For this review, take the finished solid that the model builds, in its own axes (mm). A direction names the side the tool comes from. Give positions to 0.01 mm unless a question says otherwise; leave off trailing zeros. Use a Markdown table: item, result. Add a question column.
1) Machinability: for faces 1 (the face through (1.972, 219.188, -129.733)), 2 (the face through (0, 118, -125)), which of the approach directions +Z, -Z, +X, -X, +Y, -Y give a long, thin tool a straight path to every point of the face, cutting with its end or side? Answer none if there is none.
2) Wall thickness on L1, parallel to Y at x = 1.15, z = -177.8; L2, parallel to Y at x = 2, z = -139.7; L3, parallel to Y at x = 2.4, z = -79: over which ranges is each line inside the solid? List them lowest first.
3) Mouldability with a two-part tool opening along Z and no side actions: class faces 3 (the face through (1.972, 212.884, -126.987)), 4 (the face through (4, 118, -125)), 5 (the face through (1.97, 225.77, -125.22)) as released by +Z, released by -Z, zero draft, split by the parting line, or undercut.
4) Clearance check with a flat-ended pin moving along its axis: P1, Ø8, axis at y = 12.7, z = -215.9, coming from the -X side. State where the tip first meets the part, or that it passes through.
5) We need section A-A on x = 2.05. Give the number of separate pieces and of enclosed holes in the cut face, then the cut area to 3 significant figures.
Autodesk Inventor part; units mm, degrees
ref_plane "YZ Plane" through (0, 0, 0) normal (1, 0, 0) x (0, 1, 0)
ref_plane "XZ Plane" through (0, 0, 0) normal (0, 1, 0) x (-1, 0, 0)
ref_plane "XY Plane" through (0, 0, 0) normal (0, 0, 1) x (1, 0, 0)
sketch "Esboço1" plane through (0, 0, 0) normal (1, 0, 0) x (0, 1, 0)
  line L0 (0, 0) -> (203.2, 0)
  line L1 (203.2, 0) -> (228.6, -254)
  line L2 (228.6, -254) -> (0, -254)
  line L3 (0, -254) -> (0, 0)
  circle A0 centre (12.7, 0) radius 2.5
  circle A1 centre (25.4, 0) radius 2.5
  circle A2 centre (38.1, 0) radius 2.5
  circle A3 centre (38.1, -12.7) radius 2.5
  circle A4 centre (25.4, -12.7) radius 2.5
  circle A5 centre (12.7, -12.7) radius 2.5
  circle A6 centre (38.1, -25.4) radius 2.5
  circle A7 centre (25.4, -25.4) radius 2.5
  circle A8 centre (12.7, -25.4) radius 2.5
  circle A9 centre (38.1, -38.1) radius 2.5
  circle A10 centre (25.4, -38.1) radius 2.5
  circle A11 centre (12.7, -38.1) radius 2.5
  circle A12 centre (38.1, -50.8) radius 2.5
  circle A13 centre (25.4, -50.8) radius 2.5
  circle A14 centre (12.7, -50.8) radius 2.5
  circle A15 centre (38.1, -63.5) radius 2.5
  circle A16 centre (25.4, -63.5) radius 2.5
  circle A17 centre (12.7, -63.5) radius 2.5
  circle A18 centre (38.1, -76.2) radius 2.5
  circle A19 centre (25.4, -76.2) radius 2.5
  circle A20 centre (12.7, -76.2) radius 2.5
  circle A21 centre (38.1, -88.9) radius 2.5
  circle A22 centre (25.4, -88.9) radius 2.5
  circle A23 centre (12.7, -88.9) radius 2.5
  circle A24 centre (38.1, -101.6) radius 2.5
  circle A25 centre (25.4, -101.6) radius 2.5
  circle A26 centre (12.7, -101.6) radius 2.5
  circle A27 centre (38.1, -114.3) radius 2.5
  circle A28 centre (25.4, -114.3) radius 2.5
  circle A29 centre (12.7, -114.3) radius 2.5
  circle A30 centre (38.1, -127) radius 2.5
  circle A31 centre (25.4, -127) radius 2.5
  circle A32 centre (12.7, -127) radius 2.5
  circle A33 centre (38.1, -139.7) radius 2.5
  circle A34 centre (25.4, -139.7) radius 2.5
  circle A35 centre (12.7, -139.7) radius 2.5
  circle A36 centre (38.1, -152.4) radius 2.5
  circle A37 centre (25.4, -152.4) radius 2.5
  circle A38 centre (12.7, -152.4) radius 2.5
  circle A39 centre (38.1, -165.1) radius 2.5
  circle A40 centre (25.4, -165.1) radius 2.5
  circle A41 centre (12.7, -165.1) radius 2.5
  circle A42 centre (38.1, -177.8) radius 2.5
  circle A43 centre (25.4, -177.8) radius 2.5
  circle A44 centre (12.7, -177.8) radius 2.5
  circle A45 centre (38.1, -190.5) radius 2.5
  circle A46 centre (25.4, -190.5) radius 2.5
  circle A47 centre (12.7, -190.5) radius 2.5
  circle A48 centre (38.1, -203.2) radius 2.5
  circle A49 centre (25.4, -203.2) radius 2.5
  circle A50 centre (12.7, -203.2) radius 2.5
  circle A51 centre (38.1, -215.9) radius 2.5
  circle A52 centre (25.4, -215.9) radius 2.5
  circle A53 centre (12.7, -215.9) radius 2.5
  circle A54 centre (38.1, -228.6) radius 2.5
  circle A55 centre (25.4, -228.6) radius 2.5
  circle A56 centre (12.7, -228.6) radius 2.5
  circle A57 centre (38.1, -241.3) radius 2.5
  circle A58 centre (25.4, -241.3) radius 2.5
  circle A59 centre (12.7, -241.3) radius 2.5
  circle A60 centre (38.1, -254) radius 2.5
  circle A61 centre (25.4, -254) radius 2.5
  circle A62 centre (12.7, -254) radius 2.5
  circle A63 centre (203.4985, -2.9851) radius 3
  circle A64 centre (204.0955, -8.9553) radius 3
  circle A65 centre (204.6926, -14.9256) radius 3
  circle A66 centre (205.2896, -20.8958) radius 3
  circle A67 centre (205.8866, -26.866) radius 3
  circle A68 centre (206.4836, -32.8362) radius 3
  circle A69 centre (207.0806, -38.8065) radius 3
  circle A70 centre (207.6777, -44.7767) radius 3
  circle A71 centre (208.2747, -50.7469) radius 3
  circle A72 centre (208.8717, -56.7171) radius 3
  circle A73 centre (209.4687, -62.6873) radius 3
  circle A74 centre (210.0658, -68.6576) radius 3
  circle A75 centre (210.6628, -74.6278) radius 3
  circle A76 centre (211.2598, -80.598) radius 3
  circle A77 centre (211.8568, -86.5682) radius 3
  circle A78 centre (212.4538, -92.5385) radius 3
  circle A79 centre (213.0509, -98.5087) radius 3
  circle A80 centre (213.6479, -104.4789) radius 3
  circle A81 centre (214.2449, -110.4491) radius 3
  circle A82 centre (214.8419, -116.4194) radius 3
  circle A83 centre (215.439, -122.3896) radius 3
  circle A84 centre (216.036, -128.3598) radius 3
  circle A85 centre (216.633, -134.33) radius 3
  circle A86 centre (217.23, -140.3002) radius 3
  circle A87 centre (217.827, -146.2705) radius 3
  circle A88 centre (218.4241, -152.2407) radius 3
  circle A89 centre (219.0211, -158.2109) radius 3
  circle A90 centre (219.6181, -164.1811) radius 3
  circle A91 centre (220.2151, -170.1514) radius 3
  circle A92 centre (220.8122, -176.1216) radius 3
  circle A93 centre (221.4092, -182.0918) radius 3
  circle A94 centre (222.0062, -188.062) radius 3
  circle A95 centre (222.6032, -194.0323) radius 3
  circle A96 centre (223.2002, -200.0025) radius 3
  circle A97 centre (223.7973, -205.9727) radius 3
  circle A98 centre (224.3943, -211.9429) radius 3
  circle A99 centre (224.9913, -217.9131) radius 3
  circle A100 centre (225.5883, -223.8834) radius 3
  circle A101 centre (226.1854, -229.8536) radius 3
  circle A102 centre (226.7824, -235.8238) radius 3
  circle A103 centre (227.3794, -241.794) radius 3
  circle A104 centre (227.9764, -247.7643) radius 3
  circle A105 centre (228.5734, -253.7345) radius 3
  line L4 (203.2, 0) -> (213.2499, 0)
  line L5 (213.2499, 0) -> (238.6499, -254)
  line L6 (238.6499, -254) -> (228.6, -254)
  line L7 (227.9764, -247.7643) -> (204.0955, -8.9553) construction
  line L8 (230.9615, -247.4657) -> (207.0806, -8.6568)
  line L9 (201.1104, -9.2538) -> (224.9913, -248.0628)
  arc A106 (224.9913, -248.0628) -> (230.9615, -247.4657) centre (227.9764, -247.7643) ccw
  arc A107 (207.0806, -8.6568) -> (201.1104, -9.2538) centre (204.0955, -8.9553) ccw
  point P0 (40.6, 0)
  point P1 (35.6, 0)
  point P2 (27.9, 0)
  point P3 (22.9, 0)
  point P4 (15.2, 0)
  point P5 (10.2, 0)
  point P6 (10.2, -254)
  point P7 (15.2, -254)
  point P8 (22.9, -254)
  point P9 (27.9, -254)
  point P10 (35.6, -254)
  point P11 (40.6, -254)
  point P12 (203.797, -5.9702)
  point P13 (204.394, -11.9404)
  point P14 (204.9911, -17.9107)
  point P15 (205.5881, -23.8809)
  point P16 (206.1851, -29.8511)
  point P17 (206.7821, -35.8213)
  point P18 (207.3792, -41.7916)
  point P19 (207.9762, -47.7618)
  point P20 (208.5732, -53.732)
  point P21 (209.1702, -59.7022)
  point P22 (209.7672, -65.6725)
  point P23 (210.3643, -71.6427)
  point P24 (210.9613, -77.6129)
  point P25 (211.5583, -83.5831)
  point P26 (212.1553, -89.5533)
  point P27 (212.7524, -95.5236)
  point P28 (213.3494, -101.4938)
  point P29 (213.9464, -107.464)
  point P30 (214.5434, -113.4342)
  point P31 (215.1404, -119.4045)
  point P32 (215.7375, -125.3747)
  point P33 (216.3345, -131.3449)
  point P34 (216.9315, -137.3151)
  point P35 (217.5285, -143.2854)
  point P36 (218.1256, -149.2556)
  point P37 (218.7226, -155.2258)
  point P38 (219.3196, -161.196)
  point P39 (219.9166, -167.1662)
  point P40 (220.5136, -173.1365)
  point P41 (221.1107, -179.1067)
  point P42 (221.7077, -185.0769)
  point P43 (222.3047, -191.0471)
  point P44 (222.9017, -197.0174)
  point P45 (223.4988, -202.9876)
  point P46 (224.0958, -208.9578)
  point P47 (224.6928, -214.928)
  point P48 (225.2898, -220.8983)
  point P49 (225.8868, -226.8685)
  point P50 (226.4839, -232.8387)
  point P51 (227.0809, -238.8089)
  point P52 (227.6779, -244.7791)
  point P53 (228.2749, -250.7494)
  point P54 (228.2749, -250.7494)
  point P55 (227.6779, -244.7791)
  point P56 (227.0809, -238.8089)
  point P57 (226.4839, -232.8387)
  point P58 (225.8868, -226.8685)
  point P59 (225.2898, -220.8983)
  point P60 (224.6928, -214.928)
  point P61 (224.0958, -208.9578)
  point P62 (223.4988, -202.9876)
  point P63 (222.9017, -197.0174)
  point P64 (222.3047, -191.0471)
  point P65 (221.7077, -185.0769)
  point P66 (221.1107, -179.1067)
  point P67 (220.5136, -173.1365)
  point P68 (219.9166, -167.1662)
  point P69 (219.3196, -161.196)
  point P70 (218.7226, -155.2258)
  point P71 (218.1256, -149.2556)
  point P72 (217.5285, -143.2854)
  point P73 (216.9315, -137.3151)
  point P74 (216.3345, -131.3449)
  point P75 (215.7375, -125.3747)
  point P76 (215.1404, -119.4045)
  point P77 (214.5434, -113.4342)
  point P78 (213.9464, -107.464)
  point P79 (213.3494, -101.4938)
  point P80 (212.7524, -95.5236)
  point P81 (212.1553, -89.5533)
  point P82 (211.5583, -83.5831)
  point P83 (210.9613, -77.6129)
  point P84 (210.3643, -71.6427)
  point P85 (209.7672, -65.6725)
  point P86 (209.1702, -59.7022)
  point P87 (208.5732, -53.732)
  point P88 (207.9762, -47.7618)
  point P89 (207.3792, -41.7916)
  point P90 (206.7821, -35.8213)
  point P91 (206.1851, -29.8511)
  point P92 (205.5881, -23.8809)
  point P93 (204.9911, -17.9107)
  point P94 (204.394, -11.9404)
  point P95 (203.797, -5.9702)
  point P96 (216.036, -128.3598)
  point P97 (207.0806, -8.6568)
  point P98 (224.9913, -248.0628)
  point P99 (201.1104, -9.2538)
  dimension "d16" = 6
  dimension "d0" = 254
  dimension "d1" = 228.6
  dimension "d2" = 203.2
  dimension "d3" = 5
  dimension "d4" = 12.7
  dimension "d5" = 12.7
  dimension "d6" = 12.7
  dimension "d9" = 12.7
  dimension "d19" = 6
  dimension "d26" = 252
  dimension "d27" = 10
extrude "Extrusão1" add sketch "Esboço1" along normal blind 4 contours L0 A63 A64 L9 A104 A105 L2 A60 A61 A62 L3 A0 A1 A2 | L4 A63 L1 | L1 A63 | A63 L4 L5 L6 A105 A104 L8 A64 | L6 L1 A105 | A105 L1 L2
equation "\"d5\" = d4"
properties part number "Guia - Intake"
Checked values:
| question | item | result |
|---|---|---|
| 1 | face 1 | +X, -X |
| 1 | face 2 | +Z, -Z, -X, +Y, -Y |
| 2 | L1 | 0 to 10.2, 15.2 to 22.9, 27.9 to 35.6, 40.6 to 217.97, 223.99 to 231.03 |
| 2 | L2 | 0 to 10.2, 15.2 to 22.9, 27.9 to 35.6, 40.6 to 214.16, 220.18 to 227.22 |
| 2 | L3 | 0 to 208.09, 214.11 to 221.15 |
| 3 | face 3 | undercut |
| 3 | face 4 | zero draft |
| 3 | face 5 | released by +Z |
| 4 | P1 | x = 0 |
| 5 | separate pieces | 1 |
| 5 | enclosed holes | 58 |
| 5 | area | 54,700 mm² |
